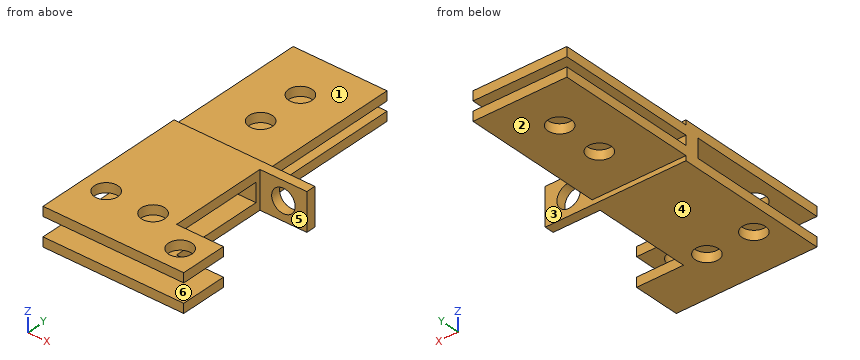
```python
from build123d import *

# Parameters (mm, degrees)
LIP_DEPTH       = 4
LIP_DEPTH_BACK  = 4
SKETCH1_W       = 20
SKETCH1_H       = 3
SIDE1_START     = 2
SKETCH1_3_W     = 20
SKETCH1_3_H     = 30
SKETCH1_3_R     = 2.5
SKETCH1_3_W_2   = 10
SKETCH1_3_H_2   = 10
SIDE1_DEPTH     = 2
SKETCH2_W       = 10
SKETCH2_H       = 8
SKETCH2_R       = 2.5
ZIP2_HOLE_DEPTH = 2
SIDE2_START     = -4
SKETCH1_4_W     = 20
SKETCH1_4_H     = 30
SKETCH1_4_R     = 2.5
SKETCH1_4_W_2   = 10
SKETCH1_4_H_2   = 10
SIDE2_DEPTH     = 2
GRABBER_START   = 1
SKETCH1_5_W     = 20
SKETCH1_5_H     = 30
SKETCH1_5_R     = 2.5
GRABBER_DEPTH   = 2
GRABBER_START_2 = -3
SKETCH1_6_W     = 20
SKETCH1_6_H     = 30
SKETCH1_6_R     = 2.5
GRABBER_2_DEPTH = 2


with BuildPart() as part:
    # Sketch1 → Lip (new, two sides: drawn at the far end of the back side and taken through both)
    with BuildSketch(Plane.XY.offset(-LIP_DEPTH_BACK)):
        with Locations((-24.8418229, 36.314477682)):
            Rectangle(SKETCH1_W, SKETCH1_H)
    extrude(amount=LIP_DEPTH + LIP_DEPTH_BACK)

    # Sketch1_3 → Side1 (add)
    # profile 1 of 2: a face of its own
    with BuildSketch(Plane.XY.offset(SIDE1_START)):
        with Locations((-24.8418229, 19.814477682)):
            Rectangle(SKETCH1_3_W, SKETCH1_3_H)
        with Locations((-29.8418229, 14.814477682)):
            Circle(SKETCH1_3_R, mode=Mode.SUBTRACT)
        with Locations((-19.8418229, 14.814477682)):
            Circle(SKETCH1_3_R, mode=Mode.SUBTRACT)
    # profile 2 of 2: a face of its own
    with BuildSketch(Plane.XY.offset(SIDE1_START)):
        with Locations((-9.8418229, 9.814477682)):
            Rectangle(SKETCH1_3_W_2, SKETCH1_3_H_2)
        with Locations((-9.8418229, 9.814477682)):
            Circle(SKETCH1_3_R, mode=Mode.SUBTRACT)
    extrude(amount=SIDE1_DEPTH)

    # Sketch2 → Zip2 Hole (add)
    with BuildSketch(Plane(origin=(0, 37.814477682, 0), x_dir=(1, 0, 0), z_dir=(0, 1, 0))):
        with Locations((-9.8418229, 0)):
            Rectangle(SKETCH2_W, SKETCH2_H)
        with Locations(Location((-9.8418229, 0, 0), (0, 0, 180))):
            Circle(SKETCH2_R, mode=Mode.SUBTRACT)
    extrude(amount=-ZIP2_HOLE_DEPTH)

    # Sketch1_4 → Side2 (add)
    # profile 1 of 2: a face of its own
    with BuildSketch(Plane.XY.offset(SIDE2_START)):
        with Locations((-24.8418229, 19.814477682)):
            Rectangle(SKETCH1_4_W, SKETCH1_4_H)
        with Locations((-29.8418229, 14.814477682)):
            Circle(SKETCH1_4_R, mode=Mode.SUBTRACT)
        with Locations((-19.8418229, 14.814477682)):
            Circle(SKETCH1_4_R, mode=Mode.SUBTRACT)
    # profile 2 of 2: a face of its own
    with BuildSketch(Plane.XY.offset(SIDE2_START)):
        with Locations((-9.8418229, 9.814477682)):
            Rectangle(SKETCH1_4_W_2, SKETCH1_4_H_2)
    extrude(amount=SIDE2_DEPTH)

    # Sketch1_5 → Grabber (add)
    with BuildSketch(Plane.XY.offset(GRABBER_START)):
        with Locations((-24.8418229, 52.814477682)):
            Rectangle(SKETCH1_5_W, SKETCH1_5_H)
        with Locations((-24.8418229, 47.814477682)):
            Circle(SKETCH1_5_R, mode=Mode.SUBTRACT)
        with Locations((-24.8418229, 57.814477682)):
            Circle(SKETCH1_5_R, mode=Mode.SUBTRACT)
    extrude(amount=GRABBER_DEPTH)

    # Sketch1_6 → Grabber 2 (add)
    with BuildSketch(Plane.XY.offset(GRABBER_START_2)):
        with Locations((-24.8418229, 52.814477682)):
            Rectangle(SKETCH1_6_W, SKETCH1_6_H)
        with Locations((-24.8418229, 47.814477682)):
            Circle(SKETCH1_6_R, mode=Mode.SUBTRACT)
        with Locations((-24.8418229, 57.814477682)):
            Circle(SKETCH1_6_R, mode=Mode.SUBTRACT)
    extrude(amount=GRABBER_2_DEPTH)


solid = part.part
```
Input: part model. Units: mm. Frame: model coordinates. Face numbers are marked on the shaded views. A direction names the side the tool comes from. Give positions to 0.01 mm unless a question says otherwise; leave off trailing zeros. Write each loop counter-clockwise with the first axis right and the second up, starting at its lowest first coordinate (ties: lowest second). Pieces come first, ordered by that corner, then holes. Notation, with made-up numbers: (-26, 48.5) - (-18, 48.5) arc R22 ccw to (-18, 87.5) - close; hole circle Ø9 at (-20, 19). An arc over 180 degrees is marked (long way). Write item = value, one per line. Start each with the question number.
1. Ray query, L1, parallel to Z at x = -31.5, y = 62; L2, parallel to Z at x = -17, y = 27.5; L3, parallel to Y at x = -5.75, z = -2.25. Return the intervals inside material, ascending.
2. Section query C-C, the plane x = -31.25. Output: boundary loops of the cut face in (y, z), then the cut area to 3 significant figures.
3. Section query B-B, the plane y = 51. Output: boundary loops of the cut face in (x, z), then the cut area to 3 significant figures.
4. First-contact query: pin 1 Ø2 at (x, z) = (-11.5, -3) entering from +Y; pin 2 Ø6 at (x, y) = (-24, 57) entering from +Z; pin 3 Ø1.6 at (y, z) = (56, -2.5) entering from +X. Flat tips, straight axial feed; report the tip coordinate or a pass-through.
5. Section query A-A, the plane z = 0. Output: boundary loops of the cut face in (x, y), then the cut area to 3 significant figures.
6. Mould query, pull axis Z, two halves, no side actions, for the marked faces 1, 2 and 3. Classes: released by +Z, released by -Z, zero draft, split by the parting line, or undercut.
7. Section query D-D, the plane y = 16.5. Output: boundary loops of the cut face in (x, z).
8. Access query for the marked faces 4, 5 and 6. Directions: +Z, -Z, +X, -X, +Y, -Y. A direction counts if a zero-diameter tool reaches every point of the face in a straight line with its end or side. Return the directions, or none.
Check sheet entries:
q1.L1 = -3 to -1, 1 to 3
q1.L2 = -4 to -2, 2 to 4
q1.L3 = 4.81 to 14.81, 35.81 to 37.81
q2.outline = (4.81, -4) - (12.75, -4) - (12.75, -2) - (4.81, -2) - close; (4.81, 2) - (12.75, 2) - (12.75, 4) - (4.81, 4) - close; (16.88, -4) - (37.81, -4) - (37.81, -3) - (67.81, -3) - (67.81, -1) - (37.81, -1) - (37.81, 1) - (67.81, 1) - (67.81, 3) - (37.81, 3) - (37.81, 4) - (16.88, 4) - (16.88, 2) - (34.81, 2) - (34.81, -2) - (16.88, -2) - close
q2.area = 247 mm2
q3.outline = (-34.84, -3) - (-14.84, -3) - (-14.84, -1) - (-34.84, -1) - close; (-34.84, 1) - (-14.84, 1) - (-14.84, 3) - (-34.84, 3) - close
q3.area = 80.0 mm2
q4.pin_1 = 37.81
q4.pin_2 = 3
q4.pin_3 = -14.84
q5.outline = (-34.84, 34.81) - (-14.84, 34.81) - (-14.84, 35.81) - (-12.34, 35.81) - (-12.34, 37.81) - (-34.84, 37.81) - close; (-7.34, 35.81) - (-4.84, 35.81) - (-4.84, 37.81) - (-7.34, 37.81) - close
q5.area = 70.0 mm2
q6.face_1 = released by +Z
q6.face_2 = released by -Z
q6.face_3 = undercut
q7.outline = (-34.84, -4) - (-31.69, -4) - (-31.69, -2) - (-34.84, -2) - close; (-34.84, 2) - (-31.69, 2) - (-31.69, 4) - (-34.84, 4) - close; (-28, -4) - (-21.69, -4) - (-21.69, -2) - (-28, -2) - close; (-28, 2) - (-21.69, 2) - (-21.69, 4) - (-28, 4) - close; (-18, -4) - (-14.84, -4) - (-14.84, -2) - (-18, -2) - close; (-18, 2) - (-14.84, 2) - (-14.84, 4) - (-18, 4) - close
q8.face_4 = -Z, +X, -X, +Y, -Y
q8.face_5 = +Z, -Z, +X
q8.face_6 = +X, -X, -Y
